CAD build for the part. Positions are in the model's coordinates, mm. A direction names the side the tool comes from. Coordinates: 2 decimals unless noted, no trailing zeros. Loops run counter-clockwise (first coordinate to the right, second up) from the corner with the lowest first, then second, coordinate; pieces in that order, holes last. Notation, with made-up numbers: (-19.75, 37.5) -> (15.25, 37.5) arc R25 cw to (15.25, 59.5) -> close; hole circle Ø10 at (87.5, 76.5). An arc over 180 degrees is marked (long way). Write item = value, one per line. Start each with the question number.
(1) Flat gauge pins, fed straight in: P1, Ø1, axis at x = 0, z = -1, coming from the -Y side; P2, Ø5, axis at y = -6, z = -1, coming from the -X side; P3, Ø1, axis at y = 0, z = 1.5, coming from the +X side; P4, Ø1.5, axis at x = -6, y = -3.5, coming from the +Z side. Where does each tip first touch, or does it go through?
(2) Band-saw the part on C-C (y = -2.5). Write the cut outline in (x, z).
(3) Band-saw the part on D-D (z = 0). Count the separate pieces of the cut face and the enclosed holes in it, and give its area (3 significant figures).
(4) Band-saw the part on A-A (x = -51.5). Write the cut outline in (y, z).
(5) Band-saw the part on B-B (y = 2.25). Write the cut outline in (x, z).
(6) Tool access for faces 1 (the face through (44, 0, 0)), 2 (the face through (-5, -1.1, 0)), 3 (the face through (-1, 1, 6)), 4 (the face through (-28.76, -5.18, -0.08)): list every direction of +Z, -Z, +X, -X, +Y, -Y with a clear straight run to the whole face (end or side of a thin tool).
(7) Drill centre lines: line 1 (Z direction, x = 45, y = 0.75); line 2 (Y direction, x = 42, z = -2.5); line 3 (Z direction, x = -51.5, y = 2.3). Where is each one in solid material? Low to high. Write a range as from..to.
```python
from build123d import *

# Parameters (mm, degrees)
SKETCH1_R                     = 1.5
BOSS_EXTRUDE1_DEPTH           = 3
SKETCH4_W                     = 3.5
SKETCH4_H                     = 12
BOSS_EXTRUDE3_DEPTH           = 10.5
SKETCH5_W                     = 2
SKETCH5_H                     = 12
BOSS_EXTRUDE4_DEPTH           = 1.1
SKETCH6_W                     = 0.2
SKETCH6_H                     = 3
BOSS_EXTRUDE5_DEPTH           = 0.5
CHAMFER1_SIZE                 = 10.5
SKETCH10_R                    = 1.5
BOSS_EXTRUDE6_DEPTH           = 2
CSK_FOR_M4_SFHCS1_D           = 4
CSK_FOR_M4_SFHCS1_DEPTH       = 30.798278762
CSK_FOR_M4_SFHCS1_CSINK_D     = 7.6
CSK_FOR_M4_SFHCS1_CSINK_ANGLE = 90
CSK_FOR_M4_SFHCS1_TIP         = 1.201721238


with BuildPart() as part:
    # Sketch1 → Boss-Extrude1 (new body)
    with BuildSketch(Plane(origin=(0, 0, 0), x_dir=(1, 0, 0), z_dir=(0, 1, 0))):
        with BuildLine():
            Line((-49, 6), (49, 6))
            ThreePointArc((49, 6), (55, 0), (49, -6))
            Line((49, -6), (-49, -6))
            ThreePointArc((-49, -6), (-55, 0), (-49, 6))
        make_face()
        with Locations(Location((-51.5, 0, 0), (0, 0, 270))):
            Circle(SKETCH1_R, mode=Mode.SUBTRACT)
        with Locations(Location((51.5, 0, 0), (0, 0, 270))):
            Circle(SKETCH1_R, mode=Mode.SUBTRACT)
    extrude(amount=BOSS_EXTRUDE1_DEPTH)

    # Sketch4 → Boss-Extrude3 (add)
    with BuildSketch(Plane.XZ):
        with Locations((-21.690023983, 0)):
            Rectangle(SKETCH4_W, SKETCH4_H)
        with Locations((21.690023983, 0)):
            Rectangle(SKETCH4_W, SKETCH4_H)
    extrude(amount=BOSS_EXTRUDE3_DEPTH)

    # Sketch5 → Boss-Extrude4 (add)
    with BuildSketch(Plane.XZ):
        with Locations((5, 0)):
            Rectangle(SKETCH5_W, SKETCH5_H)
        Rectangle(SKETCH5_W, SKETCH5_H)
        with Locations((10, 0)):
            Rectangle(SKETCH5_W, SKETCH5_H)
        with Locations((-5, 0)):
            Rectangle(SKETCH5_W, SKETCH5_H)
        with Locations((-10, 0)):
            Rectangle(SKETCH5_W, SKETCH5_H)
    extrude(amount=BOSS_EXTRUDE4_DEPTH)

    # Sketch6 → Boss-Extrude5 (add)
    with BuildSketch(Plane.XY.offset(6)):
        with Locations((48.9, 1.5)):
            Rectangle(SKETCH6_W, SKETCH6_H)
        with Locations((-48.9, 1.5)):
            Rectangle(SKETCH6_W, SKETCH6_H)
    extrude(amount=BOSS_EXTRUDE5_DEPTH)

    # Chamfer1
    chamfer1_edges = [part.edges().sort_by_distance(p)[0] for p in [
        (-23.440023983, 0, 0),
        (23.440023983, 0, 0),
    ]]
    chamfer(chamfer1_edges, length=CHAMFER1_SIZE - 0.0001)  # a hair under: the kernel refuses the full size

    # Sketch10 → Boss-Extrude6 (add)
    with BuildSketch(Plane(origin=(0, 3, 0), x_dir=(1, 0, 0), z_dir=(0, 1, 0))):
        with BuildLine():
            Line((-49, -6), (-49, -6.5))
            Line((-49, -6.5), (-48.8, -6.5))
            Line((-48.8, -6.5), (-48.8, -6))
            Line((-48.8, -6), (48.8, -6))
            Line((48.8, -6), (48.8, -6.5))
            Line((48.8, -6.5), (49, -6.5))
            Line((49, -6.5), (49, -6))
            ThreePointArc((49, -6), (55, 0), (49, 6))
            Line((49, 6), (-49, 6))
            ThreePointArc((-49, 6), (-55, 0), (-49, -6))
        make_face()
        with Locations(Location((-51.5, 0, 0), (0, 0, 270))):
            Circle(SKETCH10_R, mode=Mode.SUBTRACT)
        with Locations(Location((51.5, 0, 0), (0, 0, 270))):
            Circle(SKETCH10_R, mode=Mode.SUBTRACT)
    extrude(amount=BOSS_EXTRUDE6_DEPTH)

    # CSK for M4 SFHCS1
    with Locations(Plane(origin=(0, 5, 0), x_dir=(1, 0, 0), z_dir=(0, 1, 0))):
        with Locations((51.5, 0), (-51.5, 0)):
            CounterSinkHole(CSK_FOR_M4_SFHCS1_D / 2, CSK_FOR_M4_SFHCS1_CSINK_D / 2, depth=CSK_FOR_M4_SFHCS1_DEPTH, counter_sink_angle=CSK_FOR_M4_SFHCS1_CSINK_ANGLE)
            with Locations((0, 0, -(CSK_FOR_M4_SFHCS1_DEPTH + CSK_FOR_M4_SFHCS1_TIP / 2))):  # 118° drill point
                Cone(0, CSK_FOR_M4_SFHCS1_D / 2, CSK_FOR_M4_SFHCS1_TIP, mode=Mode.SUBTRACT)


solid = part.part
```
Findings below:
q1.P1 = -1.1
q1.P2 = -30.44
q1.P3 = 54.92
q1.P4 = through
q2.outline = (-31.44, -6) -> (-19.94, -6) -> (-19.94, 6) -> (-31.44, 6) -> close; (19.94, -6) -> (31.44, -6) -> (31.44, 6) -> (19.94, 6) -> close
q3.separate_pieces = 3
q3.enclosed_holes = 0
q3.area = 698 mm²
q4.outline = (0, -5.45) -> (5, -5.45) -> (5, -3.8) -> (3.2, -2) -> (0, -2) -> close; (0, 2) -> (3.2, 2) -> (5, 3.8) -> (5, 5.45) -> (0, 5.45) -> close
q5.outline = (-49, -6) -> (49, -6) arc R6 ccw to (49, 6) -> (49, 6.5) -> (48.8, 6.5) -> (48.8, 6) -> (-48.8, 6) -> (-48.8, 6.5) -> (-49, 6.5) -> (-49, 6) arc R6 ccw to start; hole circle Ø4 at (-51.5, 0); hole circle Ø4 at (51.5, 0)
q6.face_1 = +Z, -Z, +X, -Y
q6.face_2 = +Z, -Z, -Y
q6.face_3 = +Z, +Y, -Y
q6.face_4 = +Z, -Z, -X, -Y
q7.line_1 = -6..6
q7.line_2 = 0..5
q7.line_3 = -5.45..-2, 2..5.45
